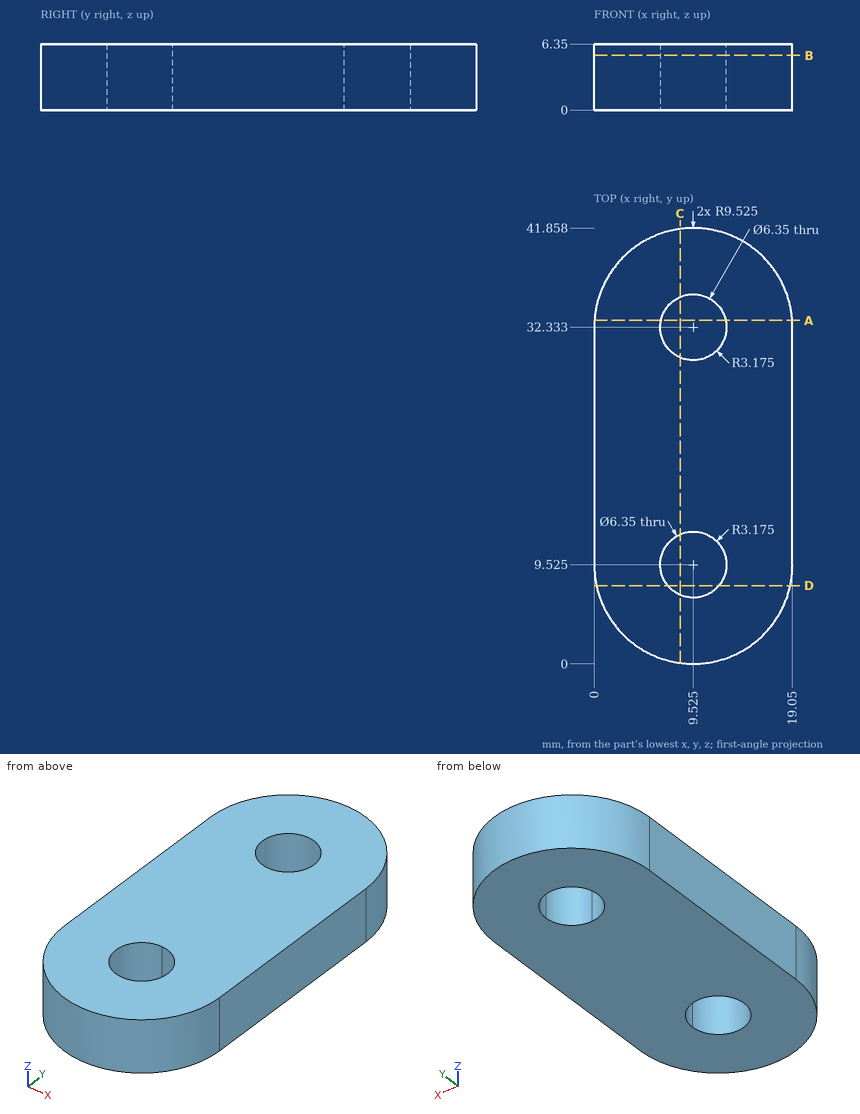
Part print with two shaded views. Sizes in mm from the minimum x, y, z corner. Coordinates: 2 decimals unless noted, no trailing zeros. Loops run counter-clockwise (first coordinate to the right, second up) from the corner with the lowest first, then second, coordinate; pieces in that order, holes last. Notation, with made-up numbers: (-7, 21.25) -> (32, 21.25) arc R21 ccw to (32, 59.25) -> close; hole circle Ø11 at (4.5, 4.5). An arc over 180 degrees is marked (long way). Answer as a JSON object with one key per item and string values.
Q1. Probe probe 1 along Y at (x, z) = (7.5, 3.75); probe 2 along Y at (x, z) = (7, 5.5); probe 3 along X at (y, z) = (10.5, 4.5). List the from-to ranges inside material, lowest first.
Report:
{"probe 1": "y = 0.22 to 7.08, 11.97 to 29.89, 34.78 to 41.64", "probe 2": "y = 0.34 to 7.6, 11.45 to 30.41, 34.26 to 41.52", "probe 3": "x = 0 to 6.5, 12.55 to 19.05"}
Q2. Cut at B-B (z = 5.25). List the corners of the cut face in (x, y) (3 decimals).
Report:
{"outline": "(0, 9.525) arc R9.525 ccw to (19.05, 9.525) -> (19.05, 32.333) arc R9.525 ccw to (0, 32.333) -> close; hole circle Ø6.35 at (9.525, 9.525); hole circle Ø6.35 at (9.525, 32.333)"}
Q3. Cut at C-C (x = 8.25). List the corners of the cut face in (y, z), and give its area (3 significant figures).
Report:
{"outline": "(0.09, 0) -> (6.62, 0) -> (6.62, 6.35) -> (0.09, 6.35) -> close; (12.43, 0) -> (29.43, 0) -> (29.43, 6.35) -> (12.43, 6.35) -> close; (35.24, 0) -> (41.77, 0) -> (41.77, 6.35) -> (35.24, 6.35) -> close", "area": "191 mm2"}
Q4. Flat gauge pins, fed straight in: P1, Ø1, axis at x = 3.5, z = 2.5, coming from the -Y side; P2, Ø1, axis at x = 4.5, z = 2, coming from the +Y side (1 decimal); P3, Ø1.5, axis at x = 8, z = 4.5, coming from the +Y side. Where does each tip first touch, or does it go through?
Report:
{"P1": "stops at y = 1.77", "P2": "stops at y = 40.7", "P3": "stops at y = 41.83"}
Q5. Cut at A-A (y = 33). List the corners of the cut face in (x, z).
Report:
{"outline": "(0.02, 0) -> (6.42, 0) -> (6.42, 6.35) -> (0.02, 6.35) -> close; (12.63, 0) -> (19.03, 0) -> (19.03, 6.35) -> (12.63, 6.35) -> close"}
Q6. Cut at D-D (y = 7.5). List the corners of the cut face in (x, z).
Report:
{"outline": "(0.22, 0) -> (7.08, 0) -> (7.08, 6.35) -> (0.22, 6.35) -> close; (11.97, 0) -> (18.83, 0) -> (18.83, 6.35) -> (11.97, 6.35) -> close"}
